Here's how the part is built. I have some questions about the finished solid (model axes, mm). Face numbers are marked on the shaded views. A direction names the side the tool comes from. Coordinates: 2 decimals unless noted, no trailing zeros. Write each loop counter-clockwise with the first axis right and the second up, starting at its lowest first coordinate (ties: lowest second). Pieces come first, ordered by that corner, then holes.
Item 1: If we section it at C-C (y = -13.5): Please give me the cut outline in (x, z).
Item 2: If we section it at D-D (x = 23): Please give me the cut outline in (y, z).
Item 3: If we section it at A-A (z = 5): Please give me the cut outline in (x, y).
Item 4: If we section it at B-B (x = 0): Please give me the cut outline in (y, z).
Item 5: We'd pull the mould along X, two halves only. Please class the marked faces 5, 6 and 7: +X half, -X half, draft (parallel to the pull), parting line (faces both ways), or undercut.
Item 6: For the marked faces 1, 2, 3 and 4, which set-ups out of +Z, -Z, +X, -X, +Y, -Y let a thin tool reach every point of the face, with its end or its side?
Item 7: If I drill on line 1 (Y direction, x = 24, z = 7.75); line 2 (Y direction, x = -13, z = 3.25); line 3 (X direction, y = 10, z = 0.5), over which ranges is the centre line in solid material (lowest first)?
Item 8: I'm going to push flat-ended pins straight in: pin 1 Ø3.5 at (x, y) = (-13, 7.5) entering from +Z; pin 2 Ø1 at (y, z) = (15.5, 2) entering from -X; pin 3 Ø2.5 at (x, y) = (-3.5, 20) entering from +Z; pin 4 Ø1 at (x, y) = (-2, 17) entering from -Z. Where does each tip first touch, or does it pass through?
from build123d import *

# Parameters (mm, degrees)
ESQUISSE1_R             = 1.6
ESQUISSE1_W             = 16
ESQUISSE1_H             = 30
BOSS_EXTRU_1_DEPTH      = 3
ESQUISSE2_W             = 20
ESQUISSE2_H             = 14
BOSS_EXTRU_2_DEPTH      = 7
ESQUISSE3_W             = 9.671871363
ESQUISSE3_H             = 10.2
ENL_V_MAT_EXTRU_1_DEPTH = 62.173932357
CHANFREIN1_SIZE         = 2
CHANFREIN2_SIZE         = 2.5
ESQUISSE4_R             = 1.6
ENL_V_MAT_EXTRU_2_DEPTH = 7
CONG_1_R                = 6
CHANFREIN3_SIZE         = 2.1


with BuildPart() as part:
    # Esquisse1 → Boss.-Extru.1 (new body)
    with BuildSketch(Plane.XY):
        Polygon((-12.5, 14.5), (-12.5, 22.5), (12.5, 22.5), (12.5, 14.5), (28, 14.5), (28, 0.5), (12.5, 0.5), (12.5, -22.5), (-12.5, -22.5), (-12.5, 0.5), (-28, 0.5), (-28, 14.5), align=None)
        with Locations((0, 17.5)):
            Circle(ESQUISSE1_R, mode=Mode.SUBTRACT)
        with Locations((0, -17.5)):
            Circle(ESQUISSE1_R, mode=Mode.SUBTRACT)
        Rectangle(ESQUISSE1_W, ESQUISSE1_H, mode=Mode.SUBTRACT)
    extrude(amount=BOSS_EXTRU_1_DEPTH)

    # Esquisse2 → Boss.-Extru.2 (add)
    with BuildSketch(Plane.XY.offset(3)):
        with Locations((-18, 7.5)):
            Rectangle(ESQUISSE2_W, ESQUISSE2_H)
        with Locations((18, 7.5)):
            Rectangle(ESQUISSE2_W, ESQUISSE2_H)
    extrude(amount=BOSS_EXTRU_2_DEPTH)

    # Esquisse3 → Enlèv. mat.-Extru.1 (cut, through all)
    with BuildSketch(Plane.ZY.offset(28)):
        with Locations((8.835935682, 7.5)):
            Rectangle(ESQUISSE3_W, ESQUISSE3_H)
    extrude(amount=-ENL_V_MAT_EXTRU_1_DEPTH, mode=Mode.SUBTRACT)

    # Chanfrein1
    chanfrein1_edges = [part.edges().sort_by_distance(p)[0] for p in [
        (28, 0.5, 5),
        (28, 14.5, 5),
        (-28, 0.5, 5),
        (-28, 14.5, 5),
    ]]
    chamfer(chanfrein1_edges, length=CHANFREIN1_SIZE)

    # Chanfrein2
    chanfrein2_edges = [part.edges().sort_by_distance(p)[0] for p in [
        (-17.95, 12.6, 4),
        (-17.95, 2.4, 4),
        (17.95, 12.6, 4),
        (17.95, 2.4, 4),
    ]]
    chamfer(chanfrein2_edges, length=CHANFREIN2_SIZE)

    # Esquisse4 → Enlèv. mat.-Extru.2 (cut)
    with BuildSketch(Plane(origin=(0, 0, 0), x_dir=(-1, 0, 0), z_dir=(0, 0, -1))):
        with Locations((23, 7.5)):
            Circle(ESQUISSE4_R)
        with Locations((13, 7.5)):
            Circle(ESQUISSE4_R)
        with Locations((-13, 7.5)):
            Circle(ESQUISSE4_R)
        with Locations((-23, 7.5)):
            Circle(ESQUISSE4_R)
    extrude(amount=-ENL_V_MAT_EXTRU_2_DEPTH, mode=Mode.SUBTRACT)

    # Congé1
    cong_1_edges = [part.edges().sort_by_distance(p)[0] for p in [
        (12.5, -22.5, 1.5),
        (-12.5, -22.5, 1.5),
        (-12.5, 22.5, 1.5),
        (12.5, 22.5, 1.5),
    ]]
    fillet(cong_1_edges, radius=CONG_1_R)

    # Chanfrein3
    chanfrein3_edges = [part.edges().sort_by_distance(p)[0] for p in [
        (-21.4, 7.5, 0),
        (-11.4, 7.5, 0),
        (14.6, 7.5, 0),
        (24.6, 7.5, 0),
    ]]
    chamfer(chanfrein3_edges, length=CHANFREIN3_SIZE)


solid = part.part
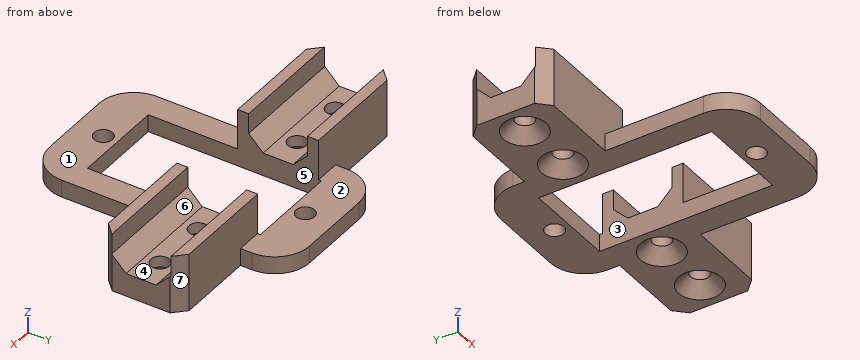
Answer list:
1. outline: (-12.5, 0) - (-8, 0) - (-8, 3) - (-12.5, 3) - close; (8, 0) - (12.5, 0) - (12.5, 3) - (8, 3) - close
2. outline: (0.5, 0) - (3.8, 0) - (5.9, 2.1) - (5.9, 4) - (4.9, 4) - (2.4, 6.5) - (2.4, 10) - (0.5, 10) - close; (9.1, 2.1) - (11.2, 0) - (14.5, 0) - (14.5, 10) - (12.6, 10) - (12.6, 6.5) - (10.1, 4) - (9.1, 4) - close
3. outline: (-28, 2.5) - (-26, 0.5) - (-8, 0.5) - (-8, 3.9) - (-28, 3.9) - close; (-28, 11.1) - (-8, 11.1) - (-8, 14.5) - (-26, 14.5) - (-28, 12.5) - close; (8, 0.5) - (26, 0.5) - (28, 2.5) - (28, 3.9) - (8, 3.9) - close; (8, 11.1) - (28, 11.1) - (28, 12.5) - (26, 14.5) - (8, 14.5) - close
4. outline: (-22.5, 0) - (-19.1, 0) - (-19.1, 3) - (-22.5, 3) - close; (-15.9, 0) - (-15, 0) - (-15, 3) - (-15.9, 3) - close; (15, 0) - (15.9, 0) - (15.9, 3) - (15, 3) - close; (19.1, 0) - (22.5, 0) - (22.5, 3) - (19.1, 3) - close
5. face 5: undercut
5. face 6: draft
5. face 7: +X half
6. face 1: +Z, +X, -X, -Y
6. face 2: +Z, +X, -X, +Y
6. face 3: +Z, -Z
6. face 4: +Z, +X, -X
7. line 1: y = 0.5 to 2.4, 12.6 to 14.5
7. line 2: y = 0.5 to 5.9, 9.1 to 14.5
7. line 3: x = -28 to -25, -21 to -15, -11 to -8, 8 to 11, 15 to 21, 25 to 28
8. pin 1: stops at z = 4
8. pin 2: stops at x = -12.5
8. pin 3: stops at z = 3
8. pin 4: stops at z = 0
